Input: part model. Units: mm. Frame: model coordinates. Coordinates: 2 decimals unless noted, no trailing zeros. Write each loop counter-clockwise with the first axis right and the second up, starting at its lowest first coordinate (ties: lowest second). Pieces come first, ordered by that corner, then holes.
from build123d import *

# Parameters (mm, degrees)
SKETCH1_W                 = 400
SKETCH1_H                 = 700
BOSS_EXTRUDE1_DEPTH       = 6.35
SKETCH2_R                 = 1.5
SKETCH2_W                 = 20
SKETCH2_H                 = 6.858
SKETCH2_R_2               = 3
CUT_EXTRUDE1_DEPTH        = 7.35
MIRROR2_COPY_1_SKETCH_R   = 1.5
MIRROR2_COPY_1_SKETCH_W   = 20
MIRROR2_COPY_1_SKETCH_H   = 6.858
MIRROR2_COPY_1_SKETCH_R_2 = 3
MIRROR2_COPY_1_DEPTH      = 7.35
CUT_EXTRUDE2_DEPTH        = 7.35
LPATTERN1_COUNT           = 5
LPATTERN1_PITCH           = 40
MIRROR3_COPY_1_DEPTH      = 7.35
MIRROR3_COPY_2_DEPTH      = 7.35
MIRROR3_COPY_3_DEPTH      = 7.35
MIRROR3_COPY_4_DEPTH      = 7.35
MIRROR3_COPY_5_DEPTH      = 7.35


with BuildPart() as part:
    # Sketch1 → Boss-Extrude1 (new body)
    with BuildSketch(Plane.XY):
        Rectangle(SKETCH1_W, SKETCH1_H)
    extrude(amount=BOSS_EXTRUDE1_DEPTH)

    # Sketch2 → Cut-Extrude1 (cut, through all)
    with BuildSketch(Plane.XY.offset(6.35)):
        with Locations((-130, 323.142)):
            Circle(SKETCH2_R)
        with Locations((-130, 330)):
            Circle(SKETCH2_R)
        with Locations((-150, 330)):
            Circle(SKETCH2_R)
        with Locations((-150, 323.142)):
            Circle(SKETCH2_R)
        with Locations((-140, 326.571)):
            Rectangle(SKETCH2_W, SKETCH2_H)
        with BuildLine():
            Line((-150, 328.5), (-150, 330))
            Line((-150, 330), (-148.5, 330))
            ThreePointArc((-148.5, 330), (-151.060660172, 331.060660172), (-150, 328.5))
        make_face()
        with BuildLine():
            Line((-148.5, 330), (-150, 330))
            Line((-150, 330), (-150, 328.5))
            ThreePointArc((-150, 328.5), (-148.939339828, 328.939339828), (-148.5, 330))
        make_face()
        with BuildLine():
            ThreePointArc((-148.5, 323.142), (-148.939339828, 324.202660172), (-150, 324.642))
            Line((-150, 324.642), (-150, 323.142))
            Line((-150, 323.142), (-148.5, 323.142))
        make_face()
        with BuildLine():
            Line((-150, 323.142), (-150, 324.642))
            ThreePointArc((-150, 324.642), (-151.060660172, 322.081339828), (-148.5, 323.142))
            Line((-148.5, 323.142), (-150, 323.142))
        make_face()
        with BuildLine():
            ThreePointArc((-128.5, 330), (-130, 331.5), (-131.5, 330))
            Line((-131.5, 330), (-130, 330))
            Line((-130, 330), (-130, 328.5))
            ThreePointArc((-130, 328.5), (-128.939339828, 328.939339828), (-128.5, 330))
        make_face()
        with BuildLine():
            Line((-130, 330), (-131.5, 330))
            ThreePointArc((-131.5, 330), (-131.060660172, 328.939339828), (-130, 328.5))
            Line((-130, 328.5), (-130, 330))
        make_face()
        with BuildLine():
            ThreePointArc((-128.5, 323.142), (-128.939339828, 324.202660172), (-130, 324.642))
            Line((-130, 324.642), (-130, 323.142))
            Line((-130, 323.142), (-131.5, 323.142))
            ThreePointArc((-131.5, 323.142), (-130, 321.642), (-128.5, 323.142))
        make_face()
        with BuildLine():
            Line((-130, 323.142), (-130, 324.642))
            ThreePointArc((-130, 324.642), (-131.060660172, 324.202660172), (-131.5, 323.142))
            Line((-131.5, 323.142), (-130, 323.142))
        make_face()
        with Locations((-180, 326.57)):
            Circle(SKETCH2_R_2)
        with Locations((-120, 326.57)):
            Circle(SKETCH2_R_2)
    cut_extrude1 = extrude(amount=-CUT_EXTRUDE1_DEPTH, mode=Mode.SUBTRACT)

    # Mirror1: Cut-Extrude1 across plane
    add(cut_extrude1.mirror(Plane.ZX), mode=Mode.SUBTRACT)

    # Mirror2: Cut-Extrude1 across plane
    add(cut_extrude1.mirror(Plane(origin=(0, 0, 0), x_dir=(0, 0, 1), z_dir=(1, 0, 0))), mode=Mode.SUBTRACT)

    # Mirror2 copy 1 sketch → Mirror2 copy 1 (cut, through all)
    with BuildSketch(Plane(origin=(0, 0, 6.35), x_dir=(-1, 0, 0), z_dir=(0, 0, 1))):
        with Locations((-130, 323.142)):
            Circle(MIRROR2_COPY_1_SKETCH_R)
        with Locations((-130, 330)):
            Circle(MIRROR2_COPY_1_SKETCH_R)
        with Locations((-150, 330)):
            Circle(MIRROR2_COPY_1_SKETCH_R)
        with Locations((-150, 323.142)):
            Circle(MIRROR2_COPY_1_SKETCH_R)
        with Locations((-140, 326.571)):
            Rectangle(MIRROR2_COPY_1_SKETCH_W, MIRROR2_COPY_1_SKETCH_H)
        with BuildLine():
            Line((-150, 328.5), (-150, 330))
            Line((-150, 330), (-148.5, 330))
            ThreePointArc((-148.5, 330), (-151.060660172, 331.060660172), (-150, 328.5))
        make_face()
        with BuildLine():
            Line((-148.5, 330), (-150, 330))
            Line((-150, 330), (-150, 328.5))
            ThreePointArc((-150, 328.5), (-148.939339828, 328.939339828), (-148.5, 330))
        make_face()
        with BuildLine():
            ThreePointArc((-148.5, 323.142), (-148.939339828, 324.202660172), (-150, 324.642))
            Line((-150, 324.642), (-150, 323.142))
            Line((-150, 323.142), (-148.5, 323.142))
        make_face()
        with BuildLine():
            Line((-150, 323.142), (-150, 324.642))
            ThreePointArc((-150, 324.642), (-151.060660172, 322.081339828), (-148.5, 323.142))
            Line((-148.5, 323.142), (-150, 323.142))
        make_face()
        with BuildLine():
            ThreePointArc((-128.5, 330), (-130, 331.5), (-131.5, 330))
            Line((-131.5, 330), (-130, 330))
            Line((-130, 330), (-130, 328.5))
            ThreePointArc((-130, 328.5), (-128.939339828, 328.939339828), (-128.5, 330))
        make_face()
        with BuildLine():
            Line((-130, 330), (-131.5, 330))
            ThreePointArc((-131.5, 330), (-131.060660172, 328.939339828), (-130, 328.5))
            Line((-130, 328.5), (-130, 330))
        make_face()
        with BuildLine():
            ThreePointArc((-128.5, 323.142), (-128.939339828, 324.202660172), (-130, 324.642))
            Line((-130, 324.642), (-130, 323.142))
            Line((-130, 323.142), (-131.5, 323.142))
            ThreePointArc((-131.5, 323.142), (-130, 321.642), (-128.5, 323.142))
        make_face()
        with BuildLine():
            Line((-130, 323.142), (-130, 324.642))
            ThreePointArc((-130, 324.642), (-131.060660172, 324.202660172), (-131.5, 323.142))
            Line((-131.5, 323.142), (-130, 323.142))
        make_face()
        with Locations((-180, 326.57)):
            Circle(MIRROR2_COPY_1_SKETCH_R_2)
        with Locations((-120, 326.57)):
            Circle(MIRROR2_COPY_1_SKETCH_R_2)
    extrude(amount=-MIRROR2_COPY_1_DEPTH, mode=Mode.SUBTRACT)

    # Sketch3 → Cut-Extrude2 (cut, through all)
    with BuildSketch(Plane.XY.offset(6.35)):
        with BuildLine():
            Line((10, 290), (10, -290))
            ThreePointArc((10, -290), (0, -300), (-10, -290))
            Line((-10, -290), (-10, 290))
            ThreePointArc((-10, 290), (0, 300), (10, 290))
        make_face()
    cut_extrude2 = extrude(amount=-CUT_EXTRUDE2_DEPTH, mode=Mode.SUBTRACT)

    # LPattern1: Cut-Extrude2 ×5
    with Locations(*[(i * LPATTERN1_PITCH, 0, 0) for i in range(1, LPATTERN1_COUNT)]):
        add(cut_extrude2, mode=Mode.SUBTRACT)

    # Mirror3 copy 1 sketch → Mirror3 copy 1 (cut, through all)
    with BuildSketch(Plane(origin=(-40, 0, 6.35), x_dir=(-1, 0, 0), z_dir=(0, 0, 1))):
        with BuildLine():
            Line((10, -290), (10, 290))
            ThreePointArc((10, 290), (0, 300), (-10, 290))
            Line((-10, 290), (-10, -290))
            ThreePointArc((-10, -290), (0, -300), (10, -290))
        make_face()
    extrude(amount=-MIRROR3_COPY_1_DEPTH, mode=Mode.SUBTRACT)

    # Mirror3 copy 2 sketch → Mirror3 copy 2 (cut, through all)
    with BuildSketch(Plane(origin=(-80, 0, 6.35), x_dir=(-1, 0, 0), z_dir=(0, 0, 1))):
        with BuildLine():
            Line((10, -290), (10, 290))
            ThreePointArc((10, 290), (0, 300), (-10, 290))
            Line((-10, 290), (-10, -290))
            ThreePointArc((-10, -290), (0, -300), (10, -290))
        make_face()
    extrude(amount=-MIRROR3_COPY_2_DEPTH, mode=Mode.SUBTRACT)

    # Mirror3 copy 3 sketch → Mirror3 copy 3 (cut, through all)
    with BuildSketch(Plane(origin=(-120, 0, 6.35), x_dir=(-1, 0, 0), z_dir=(0, 0, 1))):
        with BuildLine():
            Line((10, -290), (10, 290))
            ThreePointArc((10, 290), (0, 300), (-10, 290))
            Line((-10, 290), (-10, -290))
            ThreePointArc((-10, -290), (0, -300), (10, -290))
        make_face()
    extrude(amount=-MIRROR3_COPY_3_DEPTH, mode=Mode.SUBTRACT)

    # Mirror3 copy 4 sketch → Mirror3 copy 4 (cut, through all)
    with BuildSketch(Plane(origin=(-160, 0, 6.35), x_dir=(-1, 0, 0), z_dir=(0, 0, 1))):
        with BuildLine():
            Line((10, -290), (10, 290))
            ThreePointArc((10, 290), (0, 300), (-10, 290))
            Line((-10, 290), (-10, -290))
            ThreePointArc((-10, -290), (0, -300), (10, -290))
        make_face()
    extrude(amount=-MIRROR3_COPY_4_DEPTH, mode=Mode.SUBTRACT)

    # Mirror3 copy 5 sketch → Mirror3 copy 5 (cut, through all)
    with BuildSketch(Plane(origin=(0, 0, 6.35), x_dir=(-1, 0, 0), z_dir=(0, 0, 1))):
        with BuildLine():
            Line((10, -290), (10, 290))
            ThreePointArc((10, 290), (0, 300), (-10, 290))
            Line((-10, 290), (-10, -290))
            ThreePointArc((-10, -290), (0, -300), (10, -290))
        make_face()
    extrude(amount=-MIRROR3_COPY_5_DEPTH, mode=Mode.SUBTRACT)


solid = part.part
Item 1: Section query A-A, the plane x = 160. Return loops of the section in (y, z), then the cut area to 3 significant figures.
Item 2: Section query B-B, the plane y = -258. State how many separate pieces and enclosed holes the cut face has, then the cut area to 3 significant figures.
Item 3: Pin query (flat end, axial travel): pin 1 Ø2.5 at (x, y) = (-150, -323.142) entering from +Z. Return the tip coordinate at first contact, or that it passes through.
Item 4: Material intervals for line 1 (Y direction, x = -120, z = 1.5); line 2 (Y direction, x = -133.5, z = 3); line 3 (Y direction, x = -73.5, z = 2.5), sorted ascending.
The answers:
1. outline: (-350, 0) - (-300, 0) - (-300, 6.35) - (-350, 6.35) - close; (300, 0) - (350, 0) - (350, 6.35) - (300, 6.35) - close
1. area: 635 mm2
2. separate pieces: 10
2. enclosed holes: 0
2. area: 1,400 mm2
3. pin 1: passes through
4. line 1: y = -350 to -329.57, -323.57 to -300, 300 to 323.57, 329.57 to 350
4. line 2: y = -350 to -330, -323.14 to 323.14, 330 to 350
4. line 3: y = -350 to -297.6, 297.6 to 350
